For this review, use the dimensioned drawing (mm, ordinates from the lowest corner) and the shaded views. A direction names the side the tool comes from. Coordinates: 2 decimals unless noted, no trailing zeros. Write each loop counter-clockwise with the first axis right and the second up, starting at its lowest first coordinate (ties: lowest second). Pieces come first, ordered by that corner, then holes. Notation, with made-up numbers: (-9.5, 34) - (45.5, 34) arc R20 ccw to (45.5, 46) - close; hole circle Ø5 at (-22.5, 49). An arc over 180 degrees is marked (long way). Use one line per item in the form item = value. Start each with the question number.
1) We need section D-D (x = 74). Give the boundary of the cut face in (y, z) (3 decimals), plus the area to 3 significant figures.
2) We need section A-A (x = 50.8). Give the boundary of the cut face in (y, z) (3 decimals), plus the area to 3 significant figures.
3) We need section B-B (z = 30.5). Give the boundary of the cut face in (x, y) (3 decimals), plus the area to 3 significant figures.
4) Tool access review of the marked faces 1 and 2: name each direction out of +Z, -Z, +X, -X, +Y, -Y from which nothing blocks a thin tool from reaching the whole face with its end or side.
5) Insertion check: P1, Ø15, axis at x = 68, z = 19.5, coming from the +Y side (3 decimals); P2, Ø6, axis at x = 78.5, y = 7, coming from the +Z side (3 decimals); P3, Ø8, axis at x = 44, y = 5.5, coming from the +Z side. Each pin has a flat end and moves straight along its axis. Give the tip position at first contact, or say it passes through.
6) For L1, parallel to Y at x = 93, z = 9 (3 decimals); L2, parallel to X at y = 3, z = 25, list the stretches that pass through material, from the lowest coordinate up. Write a range as from..to.
7) We need section C-C (y = 6). Give the boundary of the cut face in (x, z) (3 decimals), plus the area to 3 significant figures.
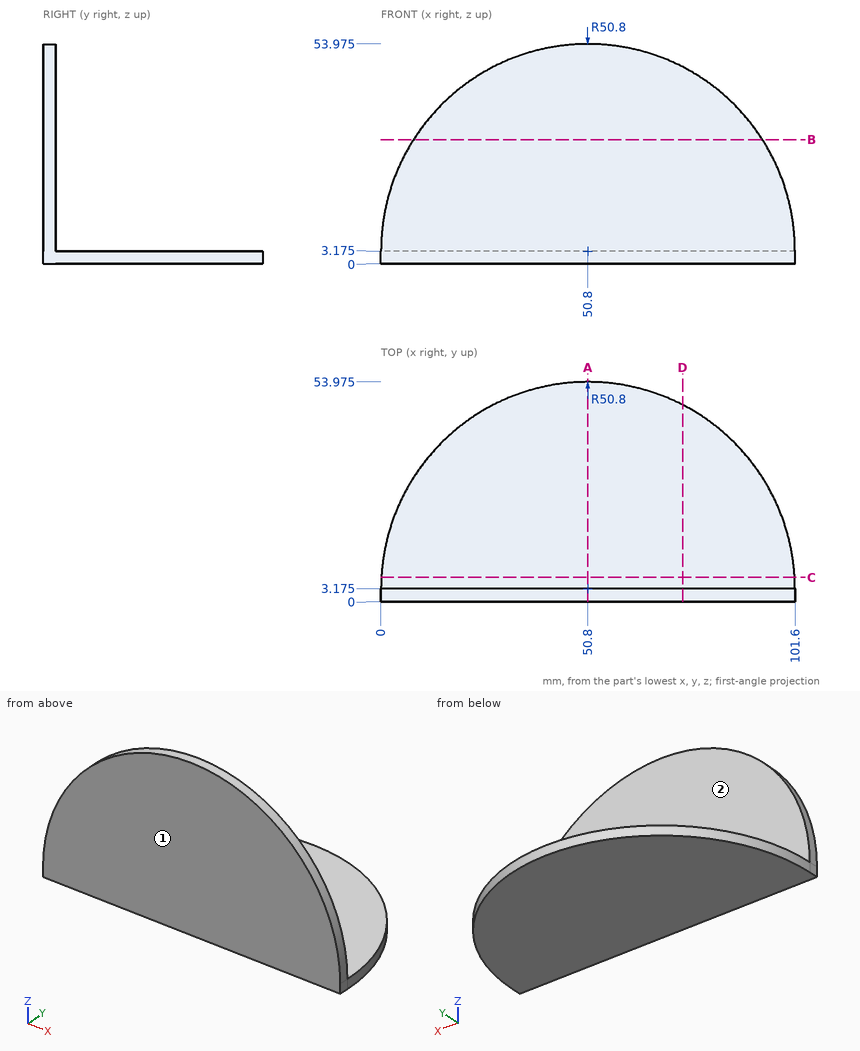
Determined:
q1.outline = (0, 0) - (48.368, 0) - (48.368, 3.175) - (3.175, 3.175) - (3.175, 48.368) - (0, 48.368) - close
q1.area = 297 mm²
q2.outline = (0, 0) - (53.975, 0) - (53.975, 3.175) - (3.175, 3.175) - (3.175, 53.975) - (0, 53.975) - close
q2.area = 333 mm²
q3.outline = (7.975, 0) - (93.625, 0) - (93.625, 3.175) - (7.975, 3.175) - close
q3.area = 272 mm²
q4.face_1 = +Z, -Z, +X, -X, -Y
q4.face_2 = +Z, +X, -X, +Y
q5.P1 = 3.175
q5.P2 = 3.175
q5.P3 = 53.85
q6.L1 = 0..3.175
q6.L2 = 4.93..96.67
q7.outline = (0.079, 0) - (101.521, 0) - (101.521, 3.175) - (0.079, 3.175) - close
q7.area = 322 mm²
